Work out the finished part from the listing and answer in its coordinate system (mm). Face numbers are marked on the shaded views. A direction names the side the tool comes from. Round coordinates to 2 decimals unless told otherwise and drop trailing zeros. Order: outer loops, then holes, each group sorted by start corner. A loop starts at its lowest first (then second) coordinate and runs counter-clockwise, first axis right, second up. Notation, with made-up numbers: (31, 56) -> (44, 56) arc R23 ccw to (44, 83) -> close; hole circle Ø2 at (4, 50). An arc over 180 degrees is marked (long way). Use one line per item in the form item = value.
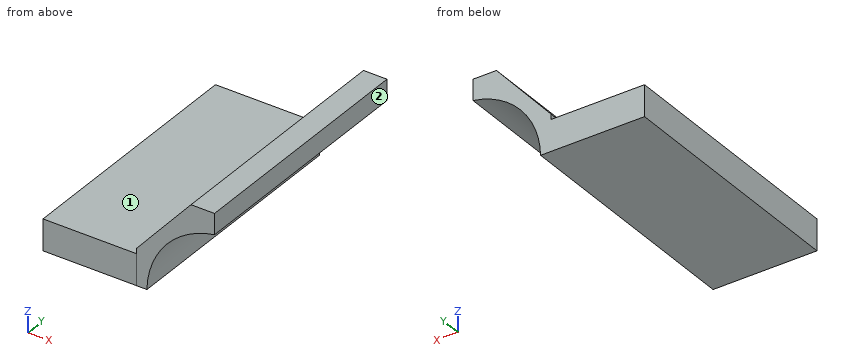
```python
from build123d import *

# Parameters (mm, degrees)
F0_W     = 57.15
F0_H     = 19.05
F1_DEPTH = 152.4000018835
F2_DEPTH = 152.4253934622


# Not quite as in the source:
# - ends of sketch curves that miss each other by under 0.0002 mm in the source are joined


with BuildPart() as f1:
    # F0 (on Front) → F1 (new body)
    with BuildSketch(Plane.XZ):
        with Locations((-23.829137, -20.6585566)):
            Rectangle(F0_W, F0_H)
    extrude(amount=F1_DEPTH)

    # F0 (on Front) → F2 (join)
    with BuildSketch(Plane.XZ):
        with BuildLine():
            Line((4.745863, -11.1335566), (4.745863, -30.1835566))
            Line((4.745863, -30.1835566), (11.100308, -30.1835566))
            ThreePointArc((11.100308, -30.1835566), (23.1263213226, 1.121334901), (52.4041128155, 17.4746845664))
            Line((52.4041128155, 17.4746845664), (52.4041116, 30.1835566))
            Line((52.4041116, 30.1835566), (38.0344934, 30.1835566))
            Line((38.0344934, 30.1835566), (4.745863, -7.9430372))
            Line((4.745863, -7.9430372), (4.745863, -11.1335566))
        make_face()
    extrude(amount=F2_DEPTH)


solid = f1.part
```
Item 1: The part is cut by section B-B, the plane x = -33. Give the vertices of the cut face in (y, z), and give its area (3 significant figures).
Findings:
outline = (-152.4, -30.18) -> (0, -30.18) -> (0, -11.13) -> (-152.4, -11.13) -> close
area = 2,900 mm^2
Item 2: For the marked faces 1 and 2, determine the directions among +Z, -Z, +X, -X, +Y, -Y from which every point of the face is accessible in a straight line to the end or side of a thin tool.
Findings:
face_1 = +Z, -X, +Y, -Y
face_2 = +Z, -Z, +X, +Y, -Y
Item 3: The part is cut by section D-D, the plane z = -1. Give the vertices of the cut face in (x, y), and give its area (3 significant figures).
Findings:
outline = (10.81, -152.43) -> (21.39, -152.43) -> (21.39, 0) -> (10.81, 0) -> close
area = 1,610 mm^2
Item 4: Flat-ended cylindrical pins translate along their axes: P1, Ø9.5, axis at x = -28.5, z = -19, coming from the -Y side; P2, Ø4, axis at y = -45, z = 10.5, coming from the +X side; P3, Ø8, axis at x = 37.5, y = -123.5, coming from the -Z side; P4, Ø2, axis at x = 11.5, y = -44.5, coming from the -Z side. Find the tip coordinate at first contact, or state that the pin passes through.
Findings:
P1 = -152.4
P2 = 37.5
P3 = 10.16
P4 = -30.18
Item 5: The part is cut by section A-A, the plane y = -121. Give the vertices of the cut face in (x, z).
Findings:
outline = (-52.4, -30.18) -> (11.1, -30.18) arc R49.26 cw to (52.4, 17.47) -> (52.4, 30.18) -> (38.03, 30.18) -> (4.75, -7.94) -> (4.75, -11.13) -> (-52.4, -11.13) -> close
Item 6: Consider line 1 along Y through (x, z) = (-9, -12); line 2 along Z through (x, y) = (-19, -41); line 3 along Z through (x, y) = (30, -105). Determine where each line is inside the solid, lowest interval first.
Findings:
line_1 = -152.4 to 0
line_2 = -30.18 to -11.13
line_3 = 7.66 to 20.98
